For this review, take the finished solid that the model builds, in its own axes (mm). Face numbers are marked on the shaded views. A direction names the side the tool comes from. Give positions to 0.01 mm unless a question says otherwise; leave off trailing zeros. Loops run counter-clockwise (first coordinate to the right, second up) from the corner with the lowest first, then second, coordinate; pieces in that order, holes last. Notation, with made-up numbers: (-26.75, -36.75) - (-21.75, -36.75) arc R21 cw to (-21.75, -31.75) - close; hole circle Ø6 at (-4.5, 31). An arc over 180 degrees is marked (long way). Answer in a Markdown table with one row per item.
```python
from build123d import *

# Parameters (mm, degrees)
SKETCH2_OUTSIDE_W  = 11.976
SKETCH2_OUTSIDE_H  = 11.976
CUT_EXTRUDE1_DEPTH = 8
SKETCH4_R          = 1.5
CUT_EXTRUDE2_DEPTH = 8
SKETCH5_W          = 1.5
SKETCH5_H          = 6.75
CUT_EXTRUDE3_DEPTH = 0.75


with BuildPart() as part:
    # Sketch1 → Revolve1 (revolve)
    with BuildSketch(Plane.XY, mode=Mode.PRIVATE) as revolve1_sk:
        with BuildLine():
            Line((1, 0), (3.175, 0))
            ThreePointArc((3.175, 0), (3.316421356, 0.058578644), (3.375, 0.2))
            Line((3.375, 0.2), (3.375, 0.839767473))
            ThreePointArc((3.375, 0.839767473), (3.351147754, 0.992356189), (3.281866736, 1.13038657))
            Line((3.281866736, 1.13038657), (2.125, 2.75))
            Line((2.125, 2.75), (2.125, 9.05))
            Line((2.125, 9.05), (2.125, 13))
            Line((2.125, 13), (1, 13))
            Line((1, 13), (1, 0))
        make_face()
    revolve(revolve1_sk.sketch.rotate(Axis((0, 13, 0), (0, -1, 0)), 90), axis=Axis((0, 13, 0), (0, -1, 0)))

    # Sketch2 outside → Cut-Extrude1 (cut)
    with BuildSketch(Plane(origin=(0, 13, 0), x_dir=(1, 0, 0), z_dir=(0, 1, 0))):
        Rectangle(SKETCH2_OUTSIDE_W, SKETCH2_OUTSIDE_H)
        Polygon((0, 2.531442277), (-2.531442277, 0), (0, -2.531442277), (2.531442277, 0), align=None, mode=Mode.SUBTRACT)
    extrude(amount=-CUT_EXTRUDE1_DEPTH, mode=Mode.SUBTRACT)

    # Boss-Extrude1 cone 1 section (through the dimple's axis) → Boss-Extrude1 (revolve)
    with BuildSketch(Plane(origin=(0, 5, 0), x_dir=(0, 0, -1), z_dir=(1, 0, 0))):
        Polygon((0, 0), (2.125, 0), (0, 5.838389516), align=None)
    revolve(axis=Axis((0, 5, 0), (0, 1, 0)))

    # Sketch4 → Cut-Extrude2 (cut)
    with BuildSketch(Plane(origin=(0, 13, 0), x_dir=(1, 0, 0), z_dir=(0, 1, 0))):
        with Locations(Location((0, 0, 0), (0, 0, 270))):
            Circle(SKETCH4_R)
    extrude(amount=-CUT_EXTRUDE2_DEPTH, mode=Mode.SUBTRACT)

    # Sketch5 → Cut-Extrude3 (cut)
    with BuildSketch(Plane.XZ):
        Rectangle(SKETCH5_W, SKETCH5_H)
    extrude(amount=-CUT_EXTRUDE3_DEPTH, mode=Mode.SUBTRACT)


solid = part.part
```
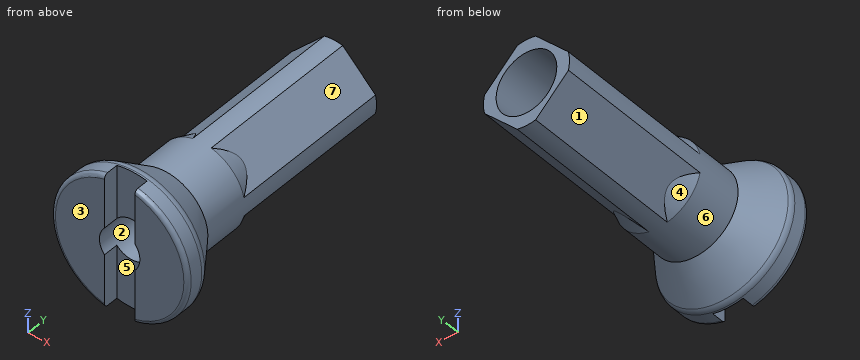
1. Clearance check with flat-ended pins moving along their axes: pin 1 (0.6 mm diameter, centred on y = 0.5, z = -2.5, fed in from +X); pin 2 (1 mm diameter, centred on x = 2.5, y = 7.5, fed in from -Z); pin 3 (0.9 mm diameter, centred on x = 0, z = -0.5, fed in from +Y); pin 4 (0.5 mm diameter, centred on x = 0, z = 2.5, fed in from -Y). State where each tip first meets the part, or that it passes through.
Values:
| item | result |
|---|---|
| pin 1 | stops at x = 2.56 |
| pin 2 | stops at z = -0.53 |
| pin 3 | passes through |
| pin 4 | stops at y = 0.75 |
2. Mouldability with a two-part tool opening along Z and no side actions: class the marked faces 1, 2 and 3 as released by +Z, released by -Z, zero draft, split by the parting line, or undercut.
Values:
| item | result |
|---|---|
| face 1 | released by -Z |
| face 2 | undercut |
| face 3 | zero draft |
3. We need section A-A, the plane x = 0. Give the boundary of the cut face in (y, z) (3 decimals).
Values:
| item | result |
|---|---|
| outline | (0.75, -3.375) - (0.84, -3.375) arc R0.5 ccw to (1.13, -3.282) - (2.75, -2.125) - (13, -2.125) - (13, -1.5) - (5, -1.5) - (5, -1) - (0.75, -1) - close; (0.75, 1) - (5, 1) - (5, 1.5) - (13, 1.5) - (13, 2.125) - (2.75, 2.125) - (1.13, 3.282) arc R0.5 ccw to (0.84, 3.375) - (0.75, 3.375) - close |
4. We need section B-B, the plane z = 0. Give the boundary of the cut face in (x, y) (3 decimals), and give its area (3 significant figures).
Values:
| item | result |
|---|---|
| outline | (-3.375, 0.2) arc R0.2 ccw to (-3.175, 0) - (-1, 0) - (-1, 5) - (-1.5, 5) - (-1.5, 13) - (-2.125, 13) - (-2.125, 2.75) - (-3.282, 1.13) arc R0.5 ccw to (-3.375, 0.84) - close; (1, 0) - (3.175, 0) arc R0.2 ccw to (3.375, 0.2) - (3.375, 0.84) arc R0.5 ccw to (3.282, 1.13) - (2.125, 2.75) - (2.125, 13) - (1.5, 13) - (1.5, 5) - (1, 5) - close |
| area | 25.9 mm^2 |
5. For the marked faces 4, 5, 6 and 7, list the 3-axis set-ups (+Z, -Z, +X, -X, +Y, -Y) from which the entire face can be reached by the end or side of a thin tool; tool diameter is ignored.
Values:
| item | result |
|---|---|
| face 4 | -Z, -X, +Y |
| face 5 | +Z, -Z, -Y |
| face 6 | +Y |
| face 7 | +Z, +X, +Y |
6. We need section C-C, the plane y = 6.5. Give the boundary of the cut face in (x, z) (3 decimals).
Values:
| item | result |
|---|---|
| outline | (-2.076, -0.456) - (-0.456, -2.076) arc R2.125 ccw to (0.456, -2.076) - (2.076, -0.456) arc R2.125 ccw to (2.076, 0.456) - (0.456, 2.076) arc R2.125 ccw to (-0.456, 2.076) - (-2.076, 0.456) arc R2.125 ccw to start; hole circle Ø3 at (0, 0) |
7. Wall thickness on line 1 (Y direction, x = -0.5, z = -1); line 2 (X direction, y = 10.75, z = 0) (3 decimals); line 3 (X direction, y = 3.8, z = 0) (3 decimals): over which ranges is each line inside the solid? List them lowest first. Write a range as [from, to].
Values:
| item | result |
|---|---|
| line 1 | y = [0.75, 5] |
| line 2 | x = [-2.125, -1.5], [1.5, 2.125] |
| line 3 | x = [-2.125, -1], [1, 2.125] |
